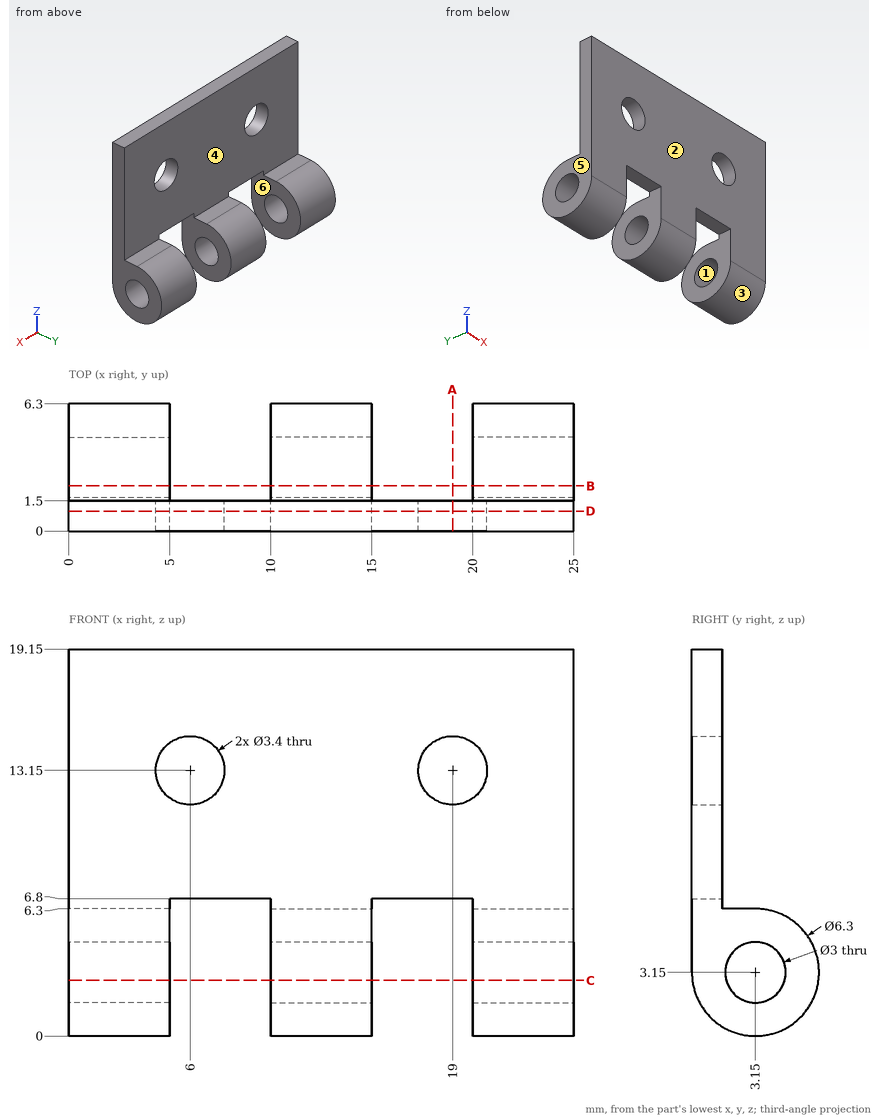
Input: dimensioned drawing with shaded views. Units: mm. Origin: part minimum x, y, z. A direction names the side the tool comes from. Coordinates: 2 decimals unless noted, no trailing zeros. Loops run counter-clockwise (first coordinate to the right, second up) from the corner with the lowest first, then second, coordinate; pieces in that order, holes last. Notation, with made-up numbers: M 74,54.25 L 107,54.25 A30 cw 107,88.25 Z; hole C 84.25,78 d3. An arc over 180 degrees is marked long. Put each result on its own line as item: value.
(1) Material intervals for probe 1 along X at (y, z) = (5, 4.75); probe 2 along X at (y, z) = (0.5, 13.15); probe 3 along Z at (x, y) = (19, 0.9), sorted ascending.
Answer sheet:
probe 1: x = 0 to 5, 10 to 15, 20 to 25
probe 2: x = 0 to 4.3, 7.7 to 17.3, 20.7 to 25
probe 3: z = 6.8 to 11.45, 14.85 to 19.15
(2) First-contact query: pin 1 (0.5 mm diameter, centred on x = 23.5, y = 2, fed in from +Z); pin 2 (1 mm diameter, centred on x = 16.5, z = 13.5, fed in from +Y); pin 3 (1.6 mm diameter, centred on x = 16.5, y = 0.5, fed in from -Z). Flat tips, straight axial feed; report the tip coordinate or a pass-through.
Answer sheet:
pin 1: stops at z = 6.3
pin 2: stops at y = 1.5
pin 3: stops at z = 6.8
(3) Draft query along Y for the marked faces 1, 2 and 3. Return one class per face: pulls with the +Y half, pulls with the -Y half, needs draft (parallel to the pull), parting line crosses it, or undercut.
Answer sheet:
face 1: undercut
face 2: pulls with the -Y half
face 3: parting line crosses it
(4) Cut plane A-A on x = 19. Return the cut outline in (y, z).
Answer sheet:
outline: M 0,6.8 L 1.5,6.8 L 1.5,11.45 L 0,11.45 Z; M 0,14.85 L 1.5,14.85 L 1.5,19.15 L 0,19.15 Z
(5) Cut plane C-C on z = 2.75. Return the cut outline in (x, y), then the cut area to 3 significant figures.
Answer sheet:
outline: M 0,0.03 L 5,0.03 L 5,1.7 L 0,1.7 Z; M 0,4.6 L 5,4.6 L 5,6.27 L 0,6.27 Z; M 10,0.03 L 15,0.03 L 15,1.7 L 10,1.7 Z; M 10,4.6 L 15,4.6 L 15,6.27 L 10,6.27 Z; M 20,0.03 L 25,0.03 L 25,1.7 L 20,1.7 Z; M 20,4.6 L 25,4.6 L 25,6.27 L 20,6.27 Z
area: 50.4 mm^2
(6) Access query for the marked faces 4, 5 and 6. Directions: +Z, -Z, +X, -X, +Y, -Y. A direction counts if a zero-diameter tool reaches every point of the face in a straight line with its end or side. Return the directions, or none.
Answer sheet:
face 4: +Z, +X, -X, +Y
face 5: +Z, -Z, -X, +Y, -Y
face 6: -Z, +Y, -Y
(7) Cut plane B-B on y = 2.25. Return the cut outline in (x, z).
Answer sheet:
outline: M 0,0.13 L 5,0.13 L 5,1.95 L 0,1.95 Z; M 0,4.35 L 5,4.35 L 5,6.3 L 0,6.3 Z; M 10,0.13 L 15,0.13 L 15,1.95 L 10,1.95 Z; M 10,4.35 L 15,4.35 L 15,6.3 L 10,6.3 Z; M 20,0.13 L 25,0.13 L 25,1.95 L 20,1.95 Z; M 20,4.35 L 25,4.35 L 25,6.3 L 20,6.3 Z
(8) Cut plane D-D on y = 1. Return the cut outline in (x, z), then the cut area to 3 significant figures.
Answer sheet:
outline: M 0,0.85 L 5,0.85 L 5,6.8 L 10,6.8 L 10,0.85 L 15,0.85 L 15,6.8 L 20,6.8 L 20,0.85 L 25,0.85 L 25,19.15 L 0,19.15 Z; hole C 6,13.15 d3.4; hole C 19,13.15 d3.4
area: 380 mm^2
